from build123d import *

# Parameters (mm, degrees)
SKETCH2_R           = 2.75
BOSS_EXTRUDE1_DEPTH = 3
SKETCH3_W           = 7
SKETCH3_H           = 5
BOSS_EXTRUDE2_DEPTH = 100
BOSS_EXTRUDE3_DEPTH = 5
SKETCH5_R           = 1.75
CUT_EXTRUDE1_DEPTH  = 5
SKETCH6_R           = 1.5
CUT_EXTRUDE2_DEPTH  = 5
SKETCH7_R           = 2.5
CUT_EXTRUDE3_DEPTH  = 7


with BuildPart() as part:
    # Sketch2 → Boss-Extrude1 (new body)
    with BuildSketch(Plane.XY):
        with BuildLine():
            Line((-20.753194099, 19.75), (-20.753194099, 16.569349275))
            ThreePointArc((-20.753194099, 16.569349275), (-23.872314522, 11.634044872), (-25.837619304, 6.136434585))
            ThreePointArc((-25.837619304, 6.136434585), (-21.386434585, -1.087619304), (-14.162380696, 3.363565415))
            ThreePointArc((-14.162380696, 3.363565415), (0, 14.556325061), (14.162380696, 3.363565415))
            ThreePointArc((14.162380696, 3.363565415), (21.386434585, -1.087619304), (25.837619304, 6.136434585))
            ThreePointArc((25.837619304, 6.136434585), (23.872314522, 11.634044872), (20.753194099, 16.569349275))
            Line((20.753194099, 16.569349275), (20.753194099, 19.75))
            Line((20.753194099, 19.75), (0, 19.75))
            Line((0, 19.75), (-20.753194099, 19.75))
        make_face()
        with Locations((-20, 4.75)):
            Circle(SKETCH2_R, mode=Mode.SUBTRACT)
        with Locations((20, 4.75)):
            Circle(SKETCH2_R, mode=Mode.SUBTRACT)
    extrude(amount=BOSS_EXTRUDE1_DEPTH)

    # Sketch3 → Boss-Extrude2 (add)
    with BuildSketch(Plane.XY.offset(3)):
        with Locations((-17.253194099, 17.25)):
            Rectangle(SKETCH3_W, SKETCH3_H)
        with Locations((17.253194099, 17.25)):
            Rectangle(SKETCH3_W, SKETCH3_H)
    extrude(amount=BOSS_EXTRUDE2_DEPTH)

    # Sketch4 → Boss-Extrude3 (add)
    with BuildSketch(Plane.XY.offset(103)):
        with BuildLine():
            Line((20.753194099, 19.75), (13.753194099, 19.75))
            Line((13.753194099, 19.75), (13.753194099, 0))
            ThreePointArc((13.753194099, 0), (0, -13.753194099), (-13.753194099, 0))
            Line((-13.753194099, 0), (-13.753194099, 19.75))
            Line((-13.753194099, 19.75), (-20.753194099, 19.75))
            Line((-20.753194099, 19.75), (-20.753194099, 0))
            ThreePointArc((-20.753194099, 0), (-16.34718685, -12.785325472), (-5, -20.141873431))
            Line((-5, -20.141873431), (-5, -23.753194099))
            Line((-5, -23.753194099), (5, -23.753194099))
            Line((5, -23.753194099), (5, -20.141873431))
            ThreePointArc((5, -20.141873431), (16.34718685, -12.785325472), (20.753194099, 0))
            Line((20.753194099, 0), (20.753194099, 19.75))
        make_face()
    extrude(amount=-BOSS_EXTRUDE3_DEPTH)

    # Sketch5 → Cut-Extrude1 (cut)
    with BuildSketch(Plane.XY.offset(103)):
        with Locations((-17.253194099, 10)):
            Circle(SKETCH5_R)
        with Locations((17.253194099, 10)):
            Circle(SKETCH5_R)
        with BuildLine():
            ThreePointArc((19.003194099, 0), (17.253194099, 1.75), (15.503194099, 0))
            Line((15.503194099, 0), (19.003194099, 0))
        make_face()
        with BuildLine():
            Line((19.003194099, 0), (15.503194099, 0))
            ThreePointArc((15.503194099, 0), (17.253194099, -1.75), (19.003194099, 0))
        make_face()
        with BuildLine():
            ThreePointArc((-19.003194099, 0), (-17.253194099, -1.75), (-15.503194099, 0))
            Line((-15.503194099, 0), (-19.003194099, 0))
        make_face()
        with BuildLine():
            Line((-19.003194099, 0), (-15.503194099, 0))
            ThreePointArc((-15.503194099, 0), (-17.253194099, 1.75), (-19.003194099, 0))
        make_face()
    extrude(amount=-CUT_EXTRUDE1_DEPTH, mode=Mode.SUBTRACT)

    # Sketch6 → Cut-Extrude2 (cut)
    with BuildSketch(Plane.XY.offset(103)):
        with Locations((-17.253194099, 16.75)):
            Circle(SKETCH6_R)
        with Locations((17.253194099, 16.75)):
            Circle(SKETCH6_R)
    extrude(amount=-CUT_EXTRUDE2_DEPTH, mode=Mode.SUBTRACT)

    # Sketch7 → Cut-Extrude3 (cut)
    with BuildSketch(Plane.XZ.offset(23.753194099)):
        with Locations((0, 103)):
            Circle(SKETCH7_R)
    extrude(amount=-CUT_EXTRUDE3_DEPTH, mode=Mode.SUBTRACT)


solid = part.part
Model file for the job. Use its own axes, mm. A direction names the side the tool comes from. Coordinates: 2 decimals unless noted, no trailing zeros. Write each loop counter-clockwise with the first axis right and the second up, starting at its lowest first coordinate (ties: lowest second). Pieces come first, ordered by that corner, then holes. Notation, with made-up numbers: (84.25, -33) -> (103.25, -33) arc R25 ccw to (103.25, -13) -> close; hole circle Ø9 at (-14.5, 80). An arc over 180 degrees is marked (long way). One line per item, written item: value. Start each with the question number.
1) Which spindle directions (+Z, -Z, +X, -X, +Y, -Y) get a long thin tool onto all of the face, cutting with end or side? Do faces 4 (the face through (17, 17, 98)), 5 (the face through (17.8, 3.1, 1.5)), 6 (the face through (-5, -22, 101)), 7 (the face through (13.753, 16, 56)). Say none if no direction does.
2) Probe probe 1 along Y at (x, z) = (-20, 1.15); probe 2 along X at (y, z) = (18, 23); probe 3 along Z at (x, y) = (12.5, 10). List the from-to ranges inside material, lowest first.
3) Slice it at B-B on x = 0. Write the cut outline in (y, z).
4) Slice it at A-A on z = 50. Write the cut outline in (x, y), then the cut area to 3 significant figures.
5) Pull direction X, two halves, no side cores. Call faces 1 (the face through (0, 16, 3)), 2 (the face through (-20.753, 16, 59)), 3 (the face through (-14, 19.75, 47)): +X half, -X half, draft (parallel to the pull), parting line (faces both ways), or undercut.
6) Flat gauge pins, fed straight in: pin 1 Ø6 at (y, z) = (13, 31) entering from -X; pin 2 Ø12 at (x, z) = (13.5, 80) entering from -Y; pin 3 Ø3 at (x, y) = (-17.25, 10) entering from +Z. Where does each tip first touch, or does it go through?
7) Slice it at D-D on y = 10. Write the cut outline in (x, z), then the cut area to 3 significant figures.
8) Slice it at C-C on y = -3. Write the cut outline in (x, z).
Answers follow:
1. face 4: +Z
1. face 5: -Z
1. face 6: +Z, -Z, -X, -Y
1. face 7: +Z, +Y
2. probe 1: -1.25 to 2, 7.5 to 19.75
2. probe 2: -20.75 to -13.75, 13.75 to 20.75
2. probe 3: 0 to 3
3. outline: (-23.75, 98) -> (-13.75, 98) -> (-13.75, 103) -> (-16.75, 103) -> (-16.75, 100.5) -> (-23.75, 100.5) -> close; (14.56, 0) -> (19.75, 0) -> (19.75, 3) -> (14.56, 3) -> close
4. outline: (-20.75, 14.75) -> (-13.75, 14.75) -> (-13.75, 19.75) -> (-20.75, 19.75) -> close; (13.75, 14.75) -> (20.75, 14.75) -> (20.75, 19.75) -> (13.75, 19.75) -> close
4. area: 70.0 mm2
5. face 1: undercut
5. face 2: -X half
5. face 3: draft
6. pin 1: x = -20.75
6. pin 2: y = 14.75
6. pin 3: z = 3
7. outline: (-24.6, 0) -> (-10.58, 0) -> (-10.58, 3) -> (-24.6, 3) -> close; (-20.75, 98) -> (-19, 98) -> (-19, 103) -> (-20.75, 103) -> close; (-15.5, 98) -> (-13.75, 98) -> (-13.75, 103) -> (-15.5, 103) -> close; (10.58, 0) -> (24.6, 0) -> (24.6, 3) -> (10.58, 3) -> close; (13.75, 98) -> (15.5, 98) -> (15.5, 103) -> (13.75, 103) -> close; (19, 98) -> (20.75, 98) -> (20.75, 103) -> (19, 103) -> close
7. area: 119 mm2
8. outline: (-20.54, 98) -> (-13.42, 98) -> (-13.42, 103) -> (-20.54, 103) -> close; (13.42, 98) -> (20.54, 98) -> (20.54, 103) -> (13.42, 103) -> close
